Verification items for the finished model (mm, model axes). A direction names the side the tool comes from. Round coordinates to 2 decimals unless told otherwise and drop trailing zeros. Write each loop counter-clockwise with the first axis right and the second up, starting at its lowest first coordinate (ties: lowest second). Pieces come first, ordered by that corner, then holes. Notation, with made-up numbers: M 51.5,21.5 L 80.5,21.5 A14 cw 80.5,29.5 Z; hole C 0,55.5 d7. An arc over 180 degrees is marked long. One line per question, with ' | ' between items. Start each with the question number.
Q1. Cross-section at C-C (x = -18.5). Record the boundary of the cut face in (y, z) (3 decimals), then the cut area to 3 significant figures.
Q2. Cross-section at A-A (y = -23.5). Record the boundary of the cut face in (x, z).
Q3. Release check for a two-part mould opening along Z. For faces 1 (the face through (-26.87, 28.57, 21.46)), 2 (the face through (5, -29.95, 13)), 3 (the face through (27, -14, 13)) record: released by +Z, released by -Z, zero draft, split by the parting line, or undercut.
Q4. Gauge pin test, flat ends, axial feed: pin 1 (1.5 mm diameter, centred on y = 20.5, z = 11, fed in from -X); pin 2 (10 mm diameter, centred on x = 14.5, z = 11, fed in from +Y). Record the tip position at first contact, or that the pin passes through.
Q5. Cross-section at D-D (y = 26.5). Record the boundary of the cut face in (x, z).
Q6. Tool access check on faces 4 (the face through (-25.7, 1, 16)), 5 (the face through (26.834, 23.546, 12.801)). Record the directions out of +Z, -Z, +X, -X, +Y, -Y that give a thin tool (end or side, any length) a straight path to the whole face; none if there is none.
Q7. Thickness scan on line 1 along X through (y, z) = (-6.5, 4); line 2 along Y through (x, z) = (-16.5, 23.75). Record the ranges inside material, lowest first. Write a range as from..to.
Q8. Cross-section at B-B (x = 0). Record the boundary of the cut face in (y, z) (3 decimals), then the cut area to 3 significant figures.
from build123d import *

# Parameters (mm, degrees)
SKETCH1_W           = 56
SKETCH1_H           = 64.5
BOSS_EXTRUDE1_DEPTH = 25.25
SKETCH2_W           = 51.4
SKETCH2_H           = 62.2
CUT_EXTRUDE1_DEPTH  = 50.614765947
FILLET1_R           = 1
FILLET3_R           = 12.75
SKETCH4_R           = 4
SKETCH4_R_2         = 1.5
CUT_EXTRUDE3_DEPTH  = 75.710999554
SKETCH5_R           = 4
SKETCH5_R_2         = 1.5
CUT_EXTRUDE4_DEPTH  = 70.380292591


with BuildPart() as part:
    # Sketch1 → Boss-Extrude1 (new body)
    with BuildSketch(Plane.XY):
        Rectangle(SKETCH1_W, SKETCH1_H)
    extrude(amount=BOSS_EXTRUDE1_DEPTH)

    # Sketch2 → Cut-Extrude1 (cut, through all)
    with BuildSketch(Plane.XY.offset(25.25)):
        with Locations((0, 1.15)):
            Rectangle(SKETCH2_W, SKETCH2_H)
    extrude(amount=-CUT_EXTRUDE1_DEPTH, mode=Mode.SUBTRACT)

    # Fillet1
    fillet1_edges = [part.edges().sort_by_distance(p)[0] for p in [
        (-25.7, -29.95, 12.625),
        (25.7, -29.95, 12.625),
        (28, -32.25, 12.625),
        (-28, -32.25, 12.625),
    ]]
    fillet(fillet1_edges, radius=FILLET1_R)

    # Fillet3
    # the kernel refuses this fillet: 12.75 mm, written as the material it takes off along each edge
    with BuildSketch(Plane(origin=(-59.875, 32.25, 25.25), x_dir=(0, 0, -1), z_dir=(1, 0, 0)), Plane(origin=(-6.175, 32.25, 25.25), x_dir=(0, 0, -1), z_dir=(1, 0, 0)), Plane(origin=(-59.875, 32.25, 0), x_dir=(0, -1, 0), z_dir=(1, 0, 0)), Plane(origin=(-6.175, 32.25, 0), x_dir=(0, -1, 0), z_dir=(1, 0, 0))) as fillet3_piece_1:
        with BuildLine():
            CenterArc((FILLET3_R, -FILLET3_R), FILLET3_R, 90, 90)
            Line((0, -FILLET3_R), (0, 0))
            Line((0, 0), (FILLET3_R, 0))
        make_face()
    extrude(amount=66.05, mode=Mode.SUBTRACT)

    # Sketch4 → Cut-Extrude3 (cut, through all)
    with BuildSketch(Plane.XZ.offset(32.25)):
        with Locations(Location((0, 12.625, 0), (0, 0, 270))):
            Circle(SKETCH4_R)
        with Locations(Location((7, 12.625, 0), (0, 0, 270))):
            Circle(SKETCH4_R_2)
        with Locations(Location((-7, 12.625, 0), (0, 0, 270))):
            Circle(SKETCH4_R_2)
        with Locations(Location((0, 5.625, 0), (0, 0, 270))):
            Circle(SKETCH4_R_2)
        with Locations(Location((0, 19.625, 0), (0, 0, 270))):
            Circle(SKETCH4_R_2)
        with Locations(Location((18.5, 12.625, 0), (0, 0, 270))):
            Circle(SKETCH4_R_2)
        with Locations(Location((-18.5, 12.625, 0), (0, 0, 270))):
            Circle(SKETCH4_R_2)
    extrude(amount=-CUT_EXTRUDE3_DEPTH, mode=Mode.SUBTRACT)

    # Sketch5 → Cut-Extrude4 (cut, through all)
    with BuildSketch(Plane.ZY.offset(28)):
        with Locations(Location((12.625, 19.54938724, 0), (0, 0, 270))):
            Circle(SKETCH5_R)
        with Locations(Location((12.625, 26.54938724, 0), (0, 0, 270))):
            Circle(SKETCH5_R_2)
        with Locations(Location((19.625, 19.54938724, 0), (0, 0, 270))):
            Circle(SKETCH5_R_2)
        with Locations(Location((12.625, 12.54938724, 0), (0, 0, 270))):
            Circle(SKETCH5_R_2)
        with Locations(Location((5.625, 19.54938724, 0), (0, 0, 270))):
            Circle(SKETCH5_R_2)
        with Locations(Location((12.625, 1.54938724, 0), (0, 0, 270))):
            Circle(SKETCH5_R_2)
        with Locations(Location((12.625, -15.45061276, 0), (0, 0, 270))):
            Circle(SKETCH5_R_2)
    extrude(amount=-CUT_EXTRUDE4_DEPTH, mode=Mode.SUBTRACT)


solid = part.part
Determined:
1) outline: M -32.25,0 L -29.95,0 L -29.95,11.125 L -32.25,11.125 Z; M -32.25,14.125 L -29.95,14.125 L -29.95,25.25 L -32.25,25.25 Z | area: 51.2 mm²
2) outline: M -28,0 L -25.7,0 L -25.7,25.25 L -28,25.25 Z; M 25.7,0 L 28,0 L 28,25.25 L 25.7,25.25 Z
3) face 1: released by +Z | face 2: zero draft | face 3: undercut
4) pin 1: passes through | pin 2: stops at y = -29.95
5) outline: M -28,2.09 L -25.7,2.09 L -25.7,11.13 L -28,11.13 Z; M -28,14.12 L -25.7,14.12 L -25.7,23.16 L -28,23.16 Z; M 25.7,2.09 L 28,2.09 L 28,11.13 L 25.7,11.13 Z; M 25.7,14.12 L 28,14.12 L 28,23.16 L 25.7,23.16 Z
6) face 4: +Z, -Z, +Y | face 5: +X, -X
7) line 1: x = -28..-25.7, 25.7..28 | line 2: y = -32.25..-29.95
8) outline: M -32.25,0 L -29.95,0 L -29.95,4.125 L -32.25,4.125 Z; M -32.25,7.125 L -29.95,7.125 L -29.95,8.625 L -32.25,8.625 Z; M -32.25,16.625 L -29.95,16.625 L -29.95,18.125 L -32.25,18.125 Z; M -32.25,21.125 L -29.95,21.125 L -29.95,25.25 L -32.25,25.25 Z | area: 25.9 mm²
